```python
from build123d import *

# Parameters (mm, degrees)
EXTRUDE_1_DEPTH     = 10
SKETCH_2_W          = 26.33
SKETCH_2_H          = 1.68
CUT_EXTRUDE_1_DEPTH = 5
CUT_EXTRUDE_2_REACH = 32.434
SKETCH_3_R          = 1.25


with BuildPart() as part:
    # 草图1 → 凸台-拉伸1 (new body)
    with BuildSketch(Plane.XY):
        Polygon((0, 0), (26.33, 0), (26.33, 6), (20.665, 11.53), (5.665, 11.53), (0, 6), align=None)
    extrude(amount=EXTRUDE_1_DEPTH)

    # 草图2 → 切除-拉伸1 (cut)
    with BuildSketch(Plane(origin=(0, 11.53, 0), x_dir=(1, 0, 0), z_dir=(0, 1, 0))):
        with Locations((13.165, -6.24)):
            Rectangle(SKETCH_2_W, SKETCH_2_H)
    extrude(amount=-CUT_EXTRUDE_1_DEPTH, mode=Mode.SUBTRACT)

    # 草图3 → 切除-拉伸2 (cut, up to next)
    with BuildSketch(Plane(origin=(0, 0, 0), x_dir=(-1, 0, 0), z_dir=(0, 0, -1)), mode=Mode.PRIVATE) as cut_extrude_2_sk1:
        with Locations((-23.565, 2.8)):
            Circle(SKETCH_3_R)
    cut_extrude_2_tool1 = extrude(cut_extrude_2_sk1.sketch, amount=-CUT_EXTRUDE_2_REACH, mode=Mode.PRIVATE) & part.part
    # 草图3 → 切除-拉伸2 (cut, up to next)
    with BuildSketch(Plane(origin=(0, 0, 0), x_dir=(-1, 0, 0), z_dir=(0, 0, -1)), mode=Mode.PRIVATE) as cut_extrude_2_sk2:
        with Locations((-2.765, 2.8)):
            Circle(SKETCH_3_R)
    cut_extrude_2_tool2 = extrude(cut_extrude_2_sk2.sketch, amount=-CUT_EXTRUDE_2_REACH, mode=Mode.PRIVATE) & part.part
    add(cut_extrude_2_tool1.solids().sort_by_distance((23.565, 2.8, 0))[0], mode=Mode.SUBTRACT)
    add(cut_extrude_2_tool2.solids().sort_by_distance((2.765, 2.8, 0))[0], mode=Mode.SUBTRACT)


solid = part.part
```
Verification items for the finished model (mm, model axes). A direction names the side the tool comes from. Round coordinates to 2 decimals unless told otherwise and drop trailing zeros. Write each loop counter-clockwise with the first axis right and the second up, starting at its lowest first coordinate (ties: lowest second). Pieces come first, ordered by that corner, then holes.
1. Section check B-B on z = 2.25. Enter the section's corners in (x, y) (3 decimals), plus the area to 3 significant figures.
2. Section check A-A on y = 2.8. Enter the section's corners in (x, z) (3 decimals).
3. Section check C-C on x = 18.5. Enter the section's corners in (y, z), plus the area to 3 significant figures.
4. Scan lines: L1, parallel to Z at x = 19.25, y = 7; L2, parallel to Y at x = 9.5, z = 6; L3, parallel to Y at x = 2, z = 5.75. Record each from-to range of solid material in increasing order.
5. Gauge pin test, flat end, axial feed: P1, Ø1, axis at x = 5, z = 6, coming from the -Y side. Record the tip position at first contact, or that the pin passes through.
6. Draft check along X on faces 3 (the cylindrical face through (24.814, 2.855, 4.93)), 4 (the flat face through (0, 3, 5)), 5 (the flat face through (13, 9, 7.08)). Enter one of: +X half, -X half, draft (parallel to the pull), parting line (faces both ways), or undercut.
7. Access from +Z, -Z, +X, -X, +Y, -Y to the whole of each face (thin tool, end or side, straight path). Record for faces 1 (the flat face through (13, 9, 5.4)), 2 (the flat face through (13, 11.53, 9)).
8. Section check D-D on y = 8. Enter the section's corners in (x, z), plus the area to 3 significant figures.
Answer:
1. outline: (0, 0) - (26.33, 0) - (26.33, 6) - (20.665, 11.53) - (5.665, 11.53) - (0, 6) - close; hole circle Ø2.5 at (2.765, 2.8); hole circle Ø2.5 at (23.565, 2.8)
1. area: 262 mm2
2. outline: (0, 0) - (1.515, 0) - (1.515, 10) - (0, 10) - close; (4.015, 0) - (22.315, 0) - (22.315, 10) - (4.015, 10) - close; (24.815, 0) - (26.33, 0) - (26.33, 10) - (24.815, 10) - close
3. outline: (0, 0) - (11.53, 0) - (11.53, 5.4) - (6.53, 5.4) - (6.53, 7.08) - (11.53, 7.08) - (11.53, 10) - (0, 10) - close
3. area: 107 mm2
4. L1: z = 0 to 5.4, 7.08 to 10
4. L2: y = 0 to 6.53
4. L3: y = 0 to 1.81, 3.79 to 6.53
5. P1: stops at y = 0
6. face 3: undercut
6. face 4: -X half
6. face 5: draft
7. face 1: +X, -X, +Y
7. face 2: +Z, -Z, +X, -X, +Y
8. outline: (2.05, 0) - (24.28, 0) - (24.28, 5.4) - (2.05, 5.4) - close; (2.05, 7.08) - (24.28, 7.08) - (24.28, 10) - (2.05, 10) - close
8. area: 185 mm2
